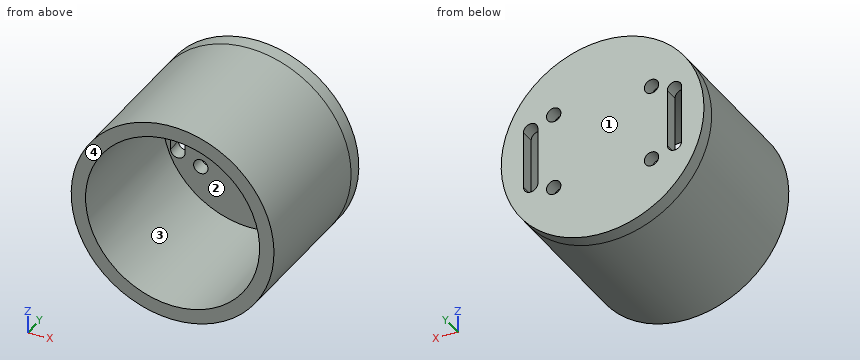
from build123d import *

# Parameters (mm, degrees)
SKETCH1_R           = 70.5
BOSS_EXTRUDE1_DEPTH = 10
SKETCH2_R           = 5
CUT_EXTRUDE1_DEPTH  = 101.202295383
BOSS_EXTRUDE2_START = 100
SKETCH3_R           = 70.5
SKETCH3_R_2         = 60.5
BOSS_EXTRUDE2_DEPTH = 100
CUT_EXTRUDE2_DEPTH  = 149.460432439


with BuildPart() as part:
    # Sketch1 → Boss-Extrude1 (new body)
    with BuildSketch(Plane(origin=(0, 0, 0), x_dir=(1, 0, 0), z_dir=(0, 1, 0))):
        with Locations(Location((0, 0, 0), (0, 0, 270))):
            Circle(SKETCH1_R)
    extrude(amount=BOSS_EXTRUDE1_DEPTH)

    # Sketch2 → Cut-Extrude1 (cut, through all)
    with BuildSketch(Plane(origin=(0, 10, 0), x_dir=(1, 0, 0), z_dir=(0, 1, 0))):
        with Locations(Location((-34, -26.5, 0), (0, 0, 270))):
            Circle(SKETCH2_R)
        with Locations(Location((34, -26.5, 0), (0, 0, 270))):
            Circle(SKETCH2_R)
        with Locations(Location((34, 26.5, 0), (0, 0, 270))):
            Circle(SKETCH2_R)
        with Locations(Location((-34, 26.5, 0), (0, 0, 270))):
            Circle(SKETCH2_R)
    extrude(amount=-CUT_EXTRUDE1_DEPTH, mode=Mode.SUBTRACT)

    # Sketch3 → Boss-Extrude2 (add)
    with BuildSketch(Plane.XZ.offset(BOSS_EXTRUDE2_START)):
        with Locations(Location((0, 0, 0), (0, 0, 270))):
            Circle(SKETCH3_R)
        with Locations(Location((0, 0, 0), (0, 0, 270))):
            Circle(SKETCH3_R_2, mode=Mode.SUBTRACT)
    extrude(amount=-BOSS_EXTRUDE2_DEPTH)

    # Sketch4 → Cut-Extrude2 (cut, through all)
    with BuildSketch(Plane(origin=(0, 10, 0), x_dir=(1, 0, 0), z_dir=(0, 1, 0))):
        with BuildLine():
            Line((55, 20), (55, -20))
            ThreePointArc((55, -20), (50, -25), (45, -20))
            Line((45, -20), (45, 20))
            ThreePointArc((45, 20), (50, 25), (55, 20))
        make_face()
    cut_extrude2 = extrude(amount=-CUT_EXTRUDE2_DEPTH, mode=Mode.SUBTRACT)

    # Mirror1: Cut-Extrude2 across plane
    add(cut_extrude2.mirror(Plane(origin=(0, 0, 0), x_dir=(0, 0, 1), z_dir=(1, 0, 0))), mode=Mode.SUBTRACT)


solid = part.part
Can you work these out from the model? Positions are in its coordinate system, mm. Face numbers are marked on the shaded views. A direction names the side the tool comes from. Round coordinates to 2 decimals unless told otherwise and drop trailing zeros. Order: outer loops, then holes, each group sorted by start corner. A loop starts at its lowest first (then second) coordinate and runs counter-clockwise, first axis right, second up. Notation, with made-up numbers: (-20.75, 36) -> (-11.75, 36) arc R28 ccw to (-11.75, 61) -> close; hole circle Ø7 at (70, -15). An arc over 180 degrees is marked (long way). Write each question's results on one line, items separated by ' | '. Start each with the question number.
Item 1: If we section it at A-A, the plane z = 0: Write out the boundary of the cut face in (x, y), then the cut area to 3 significant figures.
Item 2: Thinking about a two-plate mould opening in Z: for the marked faces 3 and 4, which applies, +Z half, -Z half, draft (parallel to the pull), parting line (faces both ways), or undercut?
Item 3: Will these pins go through, and if not, where does the flat tip stop? pin 1 (13 mm diameter, centred on x = -34, z = 26.5, fed in from -Y); pin 2 (10 mm diameter, centred on x = 27, y = -58.5, fed in from -Z); pin 3 (6 mm diameter, centred on y = -31, z = 21, fed in from +X); pin 4 (16 mm diameter, centred on x = -34, z = -26.5, fed in from +Y).
Item 4: Which directions (+Z, -Z, +X, -X, +Y, -Y) give clear straight access to the entire face, cutting with the end or side of a thin tool? Please do the marked faces 1 and 2.
Item 5: If we section it at D-D, the plane y = -10: Write out the boundary of the cut face in (x, z).
Item 6: If we section it at C-C, the plane x = 51: Write out the boundary of the cut face in (y, z).
Item 7: Please list where these lines run through material, in increasing order: L1, parallel to X at y = -40, z = 0; L2, parallel to X at y = 6, z = 26.5; L3, parallel to Y at x = 2, z = -34.5.
Item 8: If we section it at B-B, the plane x = 34: Write out the boundary of the cut face in (y, z), then the cut area to 3 significant figures.
Results:
1) outline: (-70.5, -100) -> (-60.5, -100) -> (-60.5, 0) -> (-55, 0) -> (-55, 10) -> (-70.5, 10) -> close; (-45, 0) -> (45, 0) -> (45, 10) -> (-45, 10) -> close; (55, 0) -> (60.5, 0) -> (60.5, -100) -> (70.5, -100) -> (70.5, 10) -> (55, 10) -> close | area: 3,210 mm2
2) face 3: undercut | face 4: draft
3) pin 1: stops at y = 0 | pin 2: stops at z = -66.98 | pin 3: stops at x = 68.16 | pin 4: stops at y = 10
4) face 1: +Z, -Z, +X, -X, +Y | face 2: -Y
5) outline: circle Ø141 at (0, 0); hole circle Ø121 at (0, 0)
6) outline: (-100, -48.67) -> (10, -48.67) -> (10, -24.9) -> (0, -24.9) -> (0, -32.55) -> (-100, -32.55) -> close; (-100, 32.55) -> (0, 32.55) -> (0, 24.9) -> (10, 24.9) -> (10, 48.67) -> (-100, 48.67) -> close
7) L1: x = -70.5 to -60.5, 60.5 to 70.5 | L2: x = -65.33 to -39, -29 to 29, 39 to 65.33 | L3: y = 0 to 10
8) outline: (-100, -61.76) -> (10, -61.76) -> (10, -31.5) -> (0, -31.5) -> (0, -50.04) -> (-100, -50.04) -> close; (-100, 50.04) -> (0, 50.04) -> (0, 31.5) -> (10, 31.5) -> (10, 61.76) -> (-100, 61.76) -> close; (0, -21.5) -> (10, -21.5) -> (10, 21.5) -> (0, 21.5) -> close | area: 3,380 mm2
